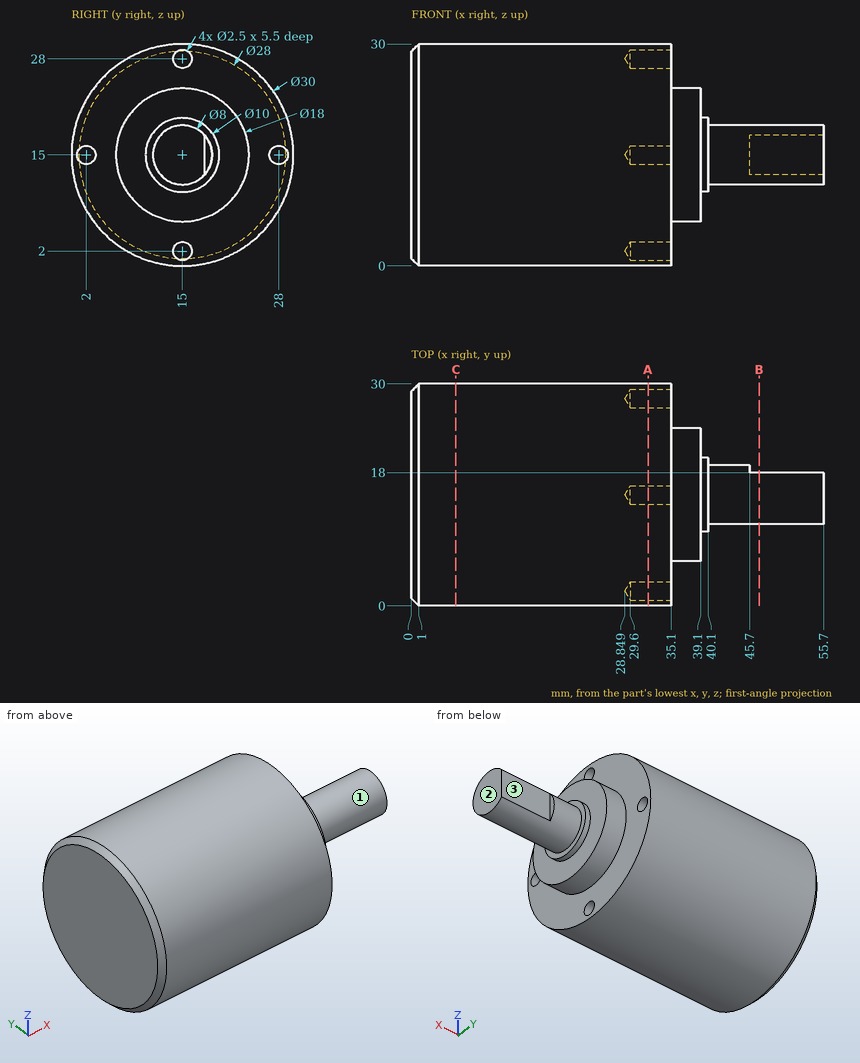
Check sheet for the drawn part. Datum: minimum x, y, z corner. Units: mm. A direction names the side the tool comes from. Give positions to 0.01 mm unless a question says otherwise; leave off trailing zeros. Write each loop counter-clockwise with the first axis right and the second up, starting at its lowest first coordinate (ties: lowest second). Pieces come first, ordered by that corner, then holes.
(1) Cross-section at A-A (x = 32). Enter the section's corners in (y, z).
(2) Gauge pin test, flat ends, axial feed: pin 1 (1.5 mm diameter, centred on x = 46.5, z = 16, fed in from -Y); pin 2 (2 mm diameter, centred on y = 28, z = 15, fed in from +X); pin 3 (1.5 mm diameter, centred on x = 16, z = 26, fed in from +Y). Record the tip position at first contact, or that the pin passes through.
(3) Cross-section at B-B (x = 47). Enter the section's corners in (y, z), plus the area to 3 significant figures.
(4) Material ranges on line 1 (Z direction, x = 32.2, y = 15); line 2 (X direction, y = 8, z = 17.75); line 3 (X direction, y = 4.25, z = 19.5), recorded low to high.
(5) Access from +Z, -Z, +X, -X, +Y, -Y to the whole of each face (thin tool, end or side, straight path). Record for the marked faces 1, 2 and 3.
(6) Cross-section at C-C (x = 6). Enter the section's corners in (y, z).
Worked out:
1. outline: circle Ø30 at (15, 15); hole circle Ø2.5 at (2, 15); hole circle Ø2.5 at (15, 2); hole circle Ø2.5 at (15, 28); hole circle Ø2.5 at (28, 15)
2. pin 1: stops at y = 11.01
2. pin 2: stops at x = 29.45
2. pin 3: stops at y = 25.95
3. outline: (18, 12.35) - (18, 17.65) arc R4 ccw (long way) to start
3. area: 46.6 mm2
4. line 1: z = 0 to 0.75, 3.25 to 26.75, 29.25 to 30
4. line 2: x = 0 to 39.1
4. line 3: x = 0 to 35.1
5. face 1: +X
5. face 2: +Z, -Z, +X, +Y, -Y
5. face 3: +Z, -Z, +X, +Y
6. outline: circle Ø30 at (15, 15)
